from build123d import *

# Parameters (mm, degrees)
SKETCH1_R           = 17.5
BOSS_EXTRUDE1_DEPTH = 3.175
SKETCH2_R           = 21
CUT_EXTRUDE1_DEPTH  = 221.006414679
CUT_EXTRUDE2_DEPTH  = 221.006414679
CIRPATTERN1_COUNT   = 3
CIRPATTERN1_ANGLE   = 240


with BuildPart() as part:
    # Sketch1 → Boss-Extrude1 (new, symmetric)
    with BuildSketch(Plane(origin=(0, 0, 0), x_dir=(1, 0, 0), z_dir=(0, 1, 0))):
        with BuildLine():
            ThreePointArc((32.5, 0), (0, 32.5), (-32.5, 0))
            Line((-32.5, 0), (-32.136420137, -4.84773151))
            ThreePointArc((-32.136420137, -4.84773151), (0, -32.5), (32.136420137, -4.84773151))
            Line((32.136420137, -4.84773151), (32.5, 0))
        make_face()
        with BuildLine():
            ThreePointArc((32.136420137, -4.84773151), (0, -32.5), (-32.136420137, -4.84773151))
            Line((-32.136420137, -4.84773151), (-17.5, -200))
            ThreePointArc((-17.5, -200), (0, -182.5), (17.5, -200))
            Line((17.5, -200), (32.136420137, -4.84773151))
        make_face()
        with Locations((0, -200)):
            Circle(SKETCH1_R)
    extrude(amount=BOSS_EXTRUDE1_DEPTH, both=True)

    # Sketch2 → Cut-Extrude1 (cut, through all)
    with BuildSketch(Plane(origin=(0, 3.175, 0), x_dir=(1, 0, 0), z_dir=(0, 1, 0))):
        with Locations(Location((0, 0, 0), (0, 0, 270))):
            Circle(SKETCH2_R)
    extrude(amount=-CUT_EXTRUDE1_DEPTH, mode=Mode.SUBTRACT)

    # Sketch4 → Cut-Extrude2 (cut, through all)
    with BuildSketch(Plane.XZ.offset(3.175)):
        with BuildLine():
            ThreePointArc((14.019152987, -18.233577529), (8.163533765, -21.502481635), (1.613875121, -22.943308547))
            ThreePointArc((1.613875121, -22.943308547), (-1.168224891, -26.14641946), (2.034886022, -28.928519473))
            ThreePointArc((2.034886022, -28.928519473), (10.293151268, -27.111824671), (17.676323332, -22.990162972))
            ThreePointArc((17.676323332, -22.990162972), (18.226030881, -18.783285078), (14.019152987, -18.233577529))
        make_face()
    cut_extrude2 = extrude(amount=-CUT_EXTRUDE2_DEPTH, mode=Mode.SUBTRACT)

    # CirPattern1: Cut-Extrude2 ×3 about axis
    cirpattern1_axis = Axis((0, 0, 0), (0, 1, 0))
    for i in range(1, CIRPATTERN1_COUNT):
        add(cut_extrude2.rotate(cirpattern1_axis, i * CIRPATTERN1_ANGLE / (CIRPATTERN1_COUNT - 1)), mode=Mode.SUBTRACT)


solid = part.part
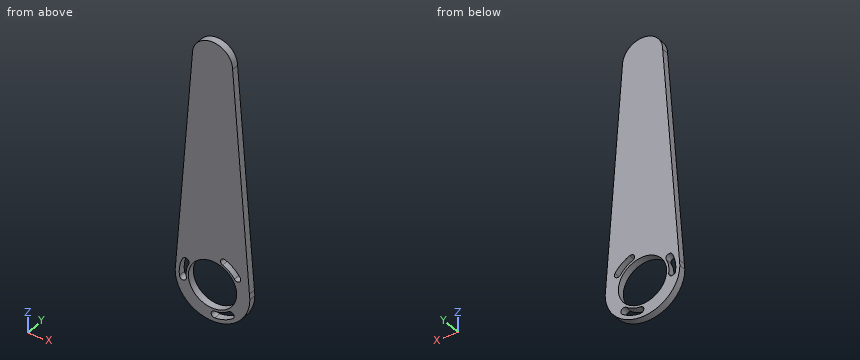
The model under review builds one solid part; all positions refer to its coordinate system, in mm. Round coordinates to 2 decimals unless told otherwise and drop trailing zeros. Write each loop counter-clockwise with the first axis right and the second up, starting at its lowest first coordinate (ties: lowest second). Pieces come first, ordered by that corner, then holes. Notation, with made-up numbers: M 39.5,30 L 53.5,30 A19 cw 53.5,65 Z; hole C 68,-11.5 d11. An arc over 180 degrees is marked long. Use a Markdown table: item, result. Add a question column.
Q1. We need section A-A, the plane y = 1.75. State the section outline as (x, z) points.
Q2. We need section C-C, the plane z = 115. State the section outline as (x, y) points (3 decimals), plus the area to 3 significant figures.
Q3. Insertion check: pin 1 (1.5 mm diameter, centred on y = -1.5, z = 132, fed in from -X); pin 2 (1 mm diameter, centred on y = -2.5, z = 156, fed in from +X); pin 3 (3 mm diameter, centred on y = -1.5, z = 78.5, fed in from +X) (3 decimals). Each pin has a flat end and moves straight along its axis. Give the tip position at first contact, or say it passes through.
Q4. We need section B-B, the plane z = 154. State the section outline as (x, y) points (3 decimals).
Q5. To check wall thickness, follow line 1 (X direction, y = 0, z = 0); line 2 (X direction, y = -2.5, z = -4); line 3 (Z direction, x = 4, y = -0.75). State the ranges of each line that lie inside material, in increasing order.
Findings below:
| question | item | result |
|---|---|---|
| 1 | outline | M -32.5,0 A32.5 ccw 32.5,0 L 17.5,200 A17.5 ccw -17.5,200 Z; hole M -28.75,-3.81 A3 ccw -22.8,-3.02 A23 cw -20.68,10.07 A3 ccw -26.07,12.7 A29 ccw Z; hole C 0,0 d42; hole M 1.61,-22.94 A3 ccw 2.03,-28.93 A29 ccw 17.68,-22.99 A3 ccw 14.02,-18.23 A23 cw Z; hole M 8.78,21.26 A23 cw 19.06,12.87 A3 ccw 24.04,16.23 A29 ccw 11.07,26.8 A3 ccw Z |
| 2 | outline | M -23.875,-3.175 L 23.875,-3.175 L 23.875,3.175 L -23.875,3.175 Z |
| 2 | area | 303 mm² |
| 3 | pin 1 | stops at x = -22.66 |
| 3 | pin 2 | stops at x = 20.84 |
| 3 | pin 3 | stops at x = 26.725 |
| 4 | outline | M -20.95,-3.175 L 20.95,-3.175 L 20.95,3.175 L -20.95,3.175 Z |
| 5 | line 1 | x = -32.5 to -29, -23 to -21, 21 to 32.5 |
| 5 | line 2 | x = -32.25 to -28.72, -22.83 to -20.62, 20.62 to 32.25 |
| 5 | line 3 | z = -32.25 to -28.72, -22.65 to -20.62, 20.62 to 217.04 |
